from build123d import *

# Parameters (mm, degrees)
F0_R     = 53.7888779042
F1_DEPTH = 271.78
F2_T     = -12
F3_R     = 7.62
F4_R     = 5.08
F5_R     = 10


with BuildPart() as f1:
    # F0 (on Top) → F1 (new body)
    with BuildSketch(Plane.XY):
        Circle(F0_R)
    extrude(amount=F1_DEPTH)

    # F2
    f2_openings = [f1.faces().sort_by_distance(p)[0] for p in [
        (0, 0, 271.78),
    ]]
    offset(amount=F2_T, openings=f2_openings)

    # F3
    f3_edges = [f1.edges().sort_by_distance(p)[0] for p in [
        (-53.788878, 0, 271.78),
    ]]
    fillet(f3_edges, radius=F3_R)

    # F4
    f4_edges = [f1.edges().sort_by_distance(p)[0] for p in [
        (-41.788878, 0, 271.78),
    ]]
    fillet(f4_edges, radius=F4_R)

    # F5
    f5_edges = [f1.edges().sort_by_distance(p)[0] for p in [
        (-53.788878, 0, 0),
        (53.788878, 0, 132.08),
        (-53.788878, 0, 264.16),
    ]]
    fillet(f5_edges, radius=F5_R)


solid = f1.part
Can you work these out from the model? Positions are in its coordinate system, mm. Coordinates: 2 decimals unless noted, no trailing zeros. Order: outer loops, then holes, each group sorted by start corner. A loop starts at its lowest first (then second) coordinate and runs counter-clockwise, first axis right, second up. Notation, with made-up numbers: M -3,9.5 L 41,9.5 A23 ccw 41,42.5 Z; hole C 35,-19.75 d1. An arc over 180 degrees is marked long. Write item = value, one per line.
(1) Suppose I cut it at A-A on z = 59.5. Please give me the cut outline in (x, y).
Results are:
outline = C 0,0 d107.58; hole C 0,0 d83.58
(2) For pin 1 Ø25 at (x, y) = (-13.5, 0) entering from +Z; pin 2 Ø2 at (y, z) = (-2, 89) entering from +X; pin 3 Ø6 at (x, z) = (41, 53.5) entering from -Y, each with a flat end and sliding along its axis, tell me the tip position at first contact or that it passes through.
Results are:
pin_1 = 12
pin_2 = 53.78
pin_3 = -38.07
(3) I need wall thicknesses on line 1 along Y through (x, z) = (0, 84); line 2 along Z through (x, y) = (-13.5, 31.5); line 3 along X through (y, z) = (32.5, 201). Which ranges of each line are inside material? Lowest first, please. Write a range as [from, to].
Results are:
line_1 = [-53.79, -41.79], [41.79, 53.79]
line_2 = [0, 12]
line_3 = [-42.86, -26.27], [26.27, 42.86]
(4) If we mould it in two halves opening along X, with no side actions, what happens to faces 1 (the face through (-11.7, -52.5, 135.3)), 2 (the face through (-1, 1, 0)), 3 (the face through (-1, 1, 12))? For each: pulls with the +X half, pulls with the -X half, needs draft (parallel to the pull), parting line crosses it, or undercut.
Results are:
face_1 = parting line crosses it
face_2 = needs draft
face_3 = undercut
